CAD build for the part. Positions are in the model's coordinates, mm. Face numbers are marked on the shaded views. A direction names the side the tool comes from. Give positions to 0.01 mm unless a question says otherwise; leave off trailing zeros. Order: outer loops, then holes, each group sorted by start corner. A loop starts at its lowest first (then second) coordinate and runs counter-clockwise, first axis right, second up.
Autodesk Inventor part; units mm, degrees
ref_plane "YZ Plane" through (0, 0, 0) normal (1, 0, 0) x (0, 1, 0)
ref_plane "XZ Plane" through (0, 0, 0) normal (0, 1, 0) x (-1, 0, 0)
ref_plane "XY Plane" through (0, 0, 0) normal (0, 0, 1) x (1, 0, 0)
sketch "Sketch1" plane through (0, 0, 0) normal (1, 0, 0) x (0, 1, 0)
  line L0 (-8, 37.75) -> (8, 37.75)
  line L1 (8, 37.75) -> (8, -37.75)
  line L2 (8, -37.75) -> (-8, -37.75)
  line L3 (-8, -37.75) -> (-8, 37.75)
  line L4 (-10, 39.75) -> (10, 39.75)
  line L5 (10, 39.75) -> (10, -39.75)
  line L6 (10, -39.75) -> (-10, -39.75)
  line L7 (-10, -39.75) -> (-10, 39.75)
  line L8 (-6.6198, 22.75) -> (6.3802, 22.75) construction
  line L9 (6.3802, 22.75) -> (6.3802, -19.25) construction
  line L10 (6.3802, -19.25) -> (-6.6198, -19.25) construction
  line L11 (-6.6198, -19.25) -> (-6.6198, 22.75) construction
  line L12 (-6.5, -21.75) -> (6.5, -21.75)
  line L13 (6.5, -21.75) -> (6.5, -29.75)
  line L14 (6.5, -29.75) -> (-6.5, -29.75)
  line L15 (-6.5, -29.75) -> (-6.5, -21.75)
  line L16 (8, 37.75) -> (-8, -37.75) construction
  line L17 (10, 39.75) -> (18, 39.75)
  line L18 (18, 39.75) -> (18, -39.75)
  line L19 (18, -39.75) -> (10, -39.75)
  line L20 (10, -39.75) -> (10, 39.75)
  line L21 (14, 29.75) -> (11, 29.75)
  line L22 (11, 29.75) -> (11, 23.75)
  line L23 (11, 23.75) -> (14, 23.75)
  line L24 (14, 23.75) -> (14, 29.75)
  line L25 (11, -20.25) -> (11, -26.25)
  line L26 (14, -26.25) -> (14, -20.25)
  line L27 (11, -26.25) -> (14, -26.25)
  line L28 (14, -20.25) -> (11, -20.25)
  point P0 (0, 0)
  point P1 (0, 0)
  point P2 (-3.5, 33.25)
  point P3 (3.5, -33.25)
  point P4 (0, 0)
  point P5 (14, 39.75)
  point P6 (12.5, 29.75)
  point P7 (10, -39.75)
  dimension "d0" = 16
  dimension "d1" = 75.5
  dimension "d2" = 4.5
  dimension "d3" = 4.5
  dimension "d4" = 2
  dimension "d5" = 4.5
  dimension "d6" = 4.5
  dimension "d7" = 13
  dimension "d8" = 42
  dimension "d9" = 15
  dimension "d10" = 13
  dimension "d11" = 8
  dimension "d12" = 1.5
  dimension "d13" = 16
  dimension "d18" = 8
  dimension "d19" = 3
  dimension "d20" = 6
  dimension "d23" = 50
  dimension "d28" = 10
  dimension "d40" = 4
extrude "Extrusion1" add sketch "Sketch1" against normal blind 3 contours L0 L1 L2 L3 | L4 L5 L6 L7
extrude "Extrusion2" add sketch "Sketch1" along normal blind 14 contours L4 L5 L6 L7
extrude "Extrusion3" add sketch "Sketch1" along normal blind 14 and the other way blind 3 contours L17 L18 L19 L5
hole "Hole1" at (0, 3.5, -33.25) at (0, -3.5, 33.25) direction (-1, 0, 0) diameter 3 end through all
fillet "Fillet1" radius 2 4 edges at (14, 14, 26.75) (14, 14, -23.25) (-3, 14, -23.25) (-3, 14, 26.75)
properties part number "rearlightMount"
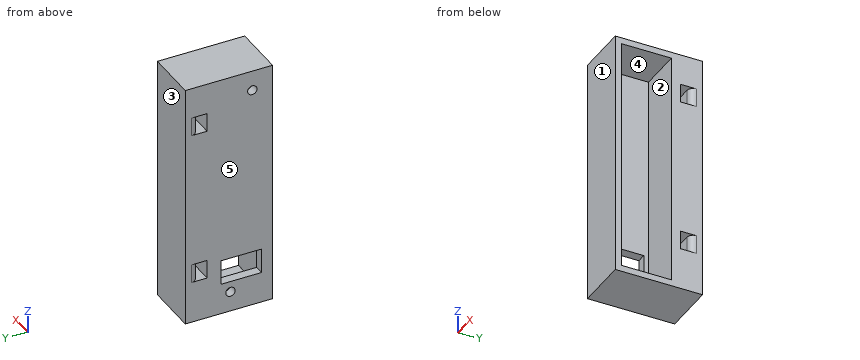
Item 1: Tool access for the marked faces 1 and 2: list every direction of +Z, -Z, +X, -X, +Y, -Y with a clear straight run to the whole face (end or side of a thin tool).
Item 2: Slice it at D-D (z = 2). Give the cut face in (x, y), and give its area (3 significant figures).
Item 3: Wall check: L1, parallel to Z at x = -0.25, y = 13.25; L2, parallel to Z at x = 11.5, y = 3.25; L3, parallel to Y at x = -1, z = -33.25. Give the ranges that are in metal, low to high.
Item 4: Slice it at B-B (y = -3.5). Give the cut face in (x, z).
Item 5: Drop flat-ended pins along their axis: pin 1 Ø2.5 at (y, z) = (3.5, -33.25) entering from +X; pin 2 Ø8 at (y, z) = (2.5, 17.5) entering from +X. Give the stop position or say it passes through.
Item 6: Slice it at A-A (z = 33.25). Give the cut face in (x, y), and give its area (3 significant figures).
Item 7: Two-plate mould, pull along Y, no slides. Class the marked faces 3, 4 and 5: released by +Y, released by -Y, zero draft, split by the parting line, or undercut.
Item 8: Slice it at C-C (x = 9.5). Give the cut face in (y, z), and give its area (3 significant figures).
A:
1. face 1: +Z, -Z, +X, -X, -Y
1. face 2: +X
2. outline: (-3, -10) - (14, -10) - (14, -8) - (0, -8) - (0, 8) - (14, 8) - (14, 18) - (-3, 18) - close
2. area: 252 mm2
3. L1: z = -39.75 to -26.25, -20.25 to 23.75, 29.75 to 39.75
3. L2: z = -39.75 to -37.75, 37.75 to 39.75
3. L3: y = -10 to 2, 5 to 18
4. outline: (-3, -39.75) - (14, -39.75) - (14, -37.75) - (0, -37.75) - (0, -29.75) - (-3, -29.75) - close; (-3, -21.75) - (0, -21.75) - (0, 31.75) - (-3, 31.75) - close; (-3, 34.75) - (0, 34.75) - (0, 37.75) - (14, 37.75) - (14, 39.75) - (-3, 39.75) - close
5. pin 1: passes through
5. pin 2: stops at x = 0
6. outline: (-3, -10) - (14, -10) - (14, -8) - (0, -8) - (0, -5) - (-3, -5) - close; (-3, -2) - (0, -2) - (0, 8) - (14, 8) - (14, 18) - (-3, 18) - close
6. area: 243 mm2
7. face 3: released by +Y
7. face 4: undercut
7. face 5: zero draft
8. outline: (-10, -39.75) - (18, -39.75) - (18, 39.75) - (-10, 39.75) - close; hole (-8, -37.75) - (8, -37.75) - (8, 37.75) - (-8, 37.75) - close; hole (11, -26.25) - (14, -26.25) - (14, -20.25) - (11, -20.25) - close; hole (11, 23.75) - (14, 23.75) - (14, 29.75) - (11, 29.75) - close
8. area: 982 mm2
